Can you work these out from the model? Positions are in its coordinate system, mm. Give positions to 0.01 mm unless a question says otherwise; leave off trailing zeros. Loops run counter-clockwise (first coordinate to the right, second up) from the corner with the lowest first, then second, coordinate; pieces in that order, holes last. Notation, with made-up numbers: (2, 72) -> (54, 72) arc R18 cw to (54, 88) -> close; hole circle Ø6 at (20.5, -13.75). An arc over 180 degrees is marked (long way). Use CSV: the item, a comma, the result in double quotes.
from build123d import *

# Parameters (mm, degrees)
BOX878_W                     = 2.2
BOX878_H                     = 20
BOX878_DEPTH                 = 28.2
BOX877_W                     = 2.2
BOX877_H                     = 20
BOX877_DEPTH                 = 28.2
COMPOUND1139_PLACEMENT_ANGLE = 90
CYLINDER2555_R               = 31
CYLINDER2555_DEPTH           = 34
CYLINDER2556_R               = 39
CYLINDER2556_DEPTH           = 3
CHAMFER090_SIZE              = 1


with BuildPart() as krychle877:
    # Box878 → Box878 (new body)
    with BuildSketch(Plane(origin=(43.9, -111, -4.1), x_dir=(1, 0, 0), z_dir=(0, 0, 1))):
        with Locations((1.1, 10)):
            Rectangle(BOX878_W, BOX878_H)
    extrude(amount=BOX878_DEPTH)


with BuildPart() as compound1139:
    # Box877 → Box877 (new body)
    with BuildSketch(Plane(origin=(-12.1, -111, -4.1), x_dir=(1, 0, 0), z_dir=(0, 0, 1))):
        with Locations((1.1, 10)):
            Rectangle(BOX877_W, BOX877_H)
    extrude(amount=BOX877_DEPTH)

    # Compound1139: union Krychle877
    add(krychle877.part)


with BuildPart() as compound1139_1:
    # Compound1139 placement: moved
    add(compound1139.part.moved(Location((-17, 10, 97))).rotate(Axis((-17, 10, 97), (1, 0, 0)), COMPOUND1139_PLACEMENT_ANGLE))


with BuildPart() as obj1:
    # Cylinder2555 → Cylinder2555 (new body)
    with BuildSketch(Plane.XY.offset(-21)):
        Circle(CYLINDER2555_R)
    extrude(amount=CYLINDER2555_DEPTH)


with BuildPart() as cut965:
    # Cylinder2556 → Cylinder2556 (new body)
    with BuildSketch(Plane.XY):
        Circle(CYLINDER2556_R)
    extrude(amount=CYLINDER2556_DEPTH)

    # Cut948: cut obj1
    add(obj1.part, mode=Mode.SUBTRACT)

    # Chamfer090
    chamfer090_edges = [cut965.edges().sort_by_distance(p)[0] for p in [
        (-39, 0, 3),
    ]]
    chamfer(chamfer090_edges, length=CHAMFER090_SIZE)


with BuildPart() as cut965_1:
    # Chamfer090 placement: moved
    add(cut965.part.moved(Location((0, 0, -8))))

    # Cut965: cut Compound1139
    add(compound1139_1.part, mode=Mode.SUBTRACT)


solid = cut965_1.part
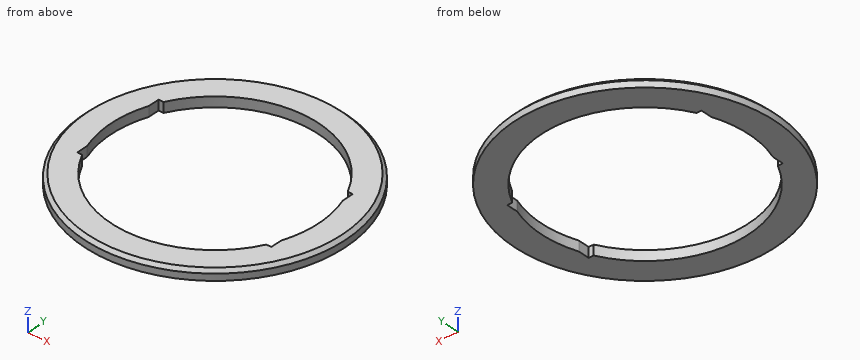
(1) If we section it at A-A, the plane x = 0: Write out the boundary of the cut face in (y, z).
Answer sheet:
outline,"(-39, -8) -> (-31, -8) -> (-31, -5) -> (-38, -5) -> (-39, -6) -> close; (31, -8) -> (39, -8) -> (39, -6) -> (38, -5) -> (31, -5) -> close"
(2) If we section it at C-C, the plane z = -6.65: Write out the boundary of the cut face in (x, y), then the cut area to 3 significant figures.
Answer sheet:
outline,"circle Ø78 at (0, 0); hole (-29.1, -14.1) -> (-27.61, -14.1) arc R31 ccw to (27.61, -14.1) -> (29.1, -14.1) -> (29.1, -10.69) arc R31 ccw to (29.1, 10.69) -> (29.1, 14.1) -> (27.61, 14.1) arc R31 ccw to (-27.61, 14.1) -> (-29.1, 14.1) -> (-29.1, 10.69) arc R31 ccw to (-29.1, -10.69) -> close"
area,"1,750 mm2"
(3) If I drill on L1, parallel to X at y = 1, z = -5.55; L2, parallel to Y at x = -13, z = -7.15; L3, parallel to X at y = 14, z = -7.4, over which ranges is the centre line in solid material (lowest first)? Write a range as from..to.
Answer sheet:
L1,"x = -38.54..-30.98, 30.98..38.54"
L2,"y = -36.77..-28.14, 28.14..36.77"
L3,"x = -36.4..-29.1, 29.1..36.4"
(4) Will these pins go through, and if not, where does the flat tip stop? pin 1 Ø1.6 at (x, z) = (-28.5, -7) entering from -Y; pin 2 Ø1.5 at (y, z) = (13, -6) entering from -X; pin 3 Ø1.6 at (x, z) = (-28, -7) entering from +Y; pin 4 Ø6 at (x, y) = (20.5, -17.5) entering from +Z.
Answer sheet:
pin 1,"stops at y = -27.45"
pin 2,"stops at x = -37.03"
pin 3,"stops at y = 27.95"
pin 4,"passes through"
